Part print with two shaded views. Sizes in mm from the minimum x, y, z corner. A direction names the side the tool comes from. Round coordinates to 2 decimals unless told otherwise and drop trailing zeros. Write each loop counter-clockwise with the first axis right and the second up, starting at its lowest first coordinate (ties: lowest second). Pieces come first, ordered by that corner, then holes. Notation, with made-up numbers: (-31.75, 66) -> (-25.75, 66) arc R22 cw to (-25.75, 88) -> close; hole circle Ø2 at (86, -1.75). An arc over 180 degrees is marked (long way). Return JSON: item names as keys, results as strings. Group by question number.
(1) Saw through at A-A (z = 17.5). List the corners of the cut face in (x, y).
(2) Tool access for the marked faces 1 and 2: list every direction of +Z, -Z, +X, -X, +Y, -Y with a clear straight run to the whole face (end or side of a thin tool).
(3) Drop a flat-ended pin along its axis: pin 1 Ø5 at (x, y) = (178.5, 13) entering from -Z. Give the stop position or say it passes through.
(4) Saw through at C-C (y = 6.5). List the corners of the cut face in (x, z).
(5) Mould opens along Y. For the marked faces 3, 4 and 5 say: +Y half, -Y half, draft (parallel to the pull), parting line (faces both ways), or undercut.
(6) Drill centre lines: L1, parallel to Y at x = 182, z = 36; L2, parallel to X at y = 6, z = 43; L3, parallel to X at y = 35.5, z = 45. Where is each one in solid material? Low to high. Write a range as from..to.
(7) Saw through at B-B (x = 87). List the corners of the cut face in (y, z), plus the area to 3 significant figures.
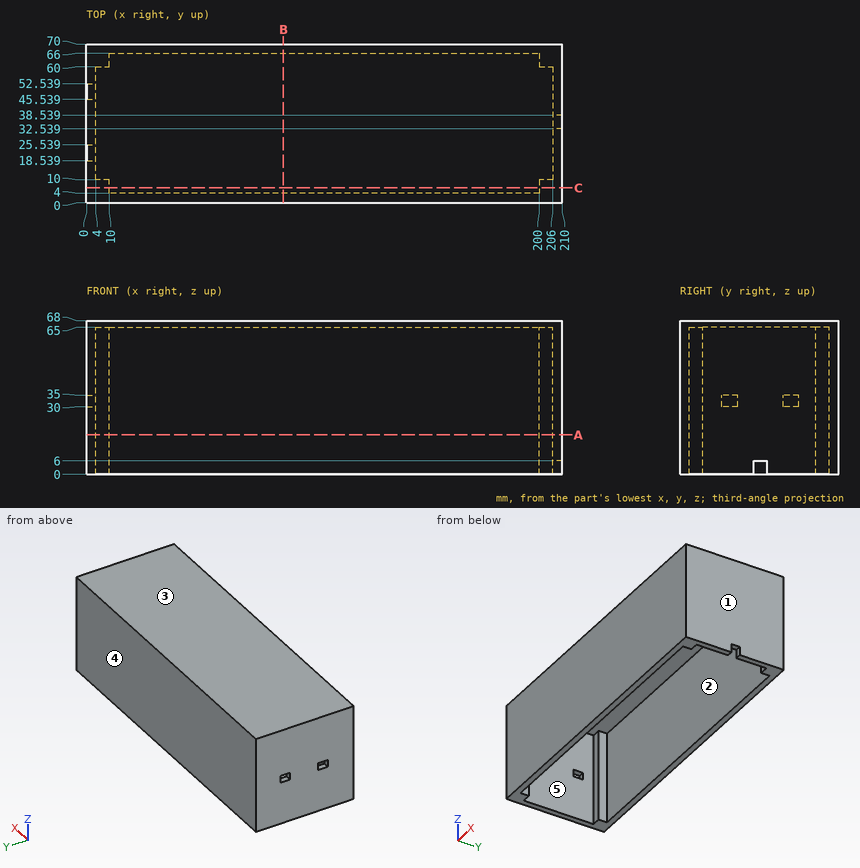
Computed values:
{
 "1": {"outline": "(0, 0) -> (210, 0) -> (210, 70) -> (0, 70) -> close; hole (4, 10) -> (10, 10) -> (10, 4) -> (200, 4) -> (200, 10) -> (206, 10) -> (206, 60) -> (200, 60) -> (200, 66) -> (10, 66) -> (10, 60) -> (4, 60) -> close"},
 "2": {"face 1": "+Z, -Z, +X, +Y, -Y", "face 2": "-Z"},
 "3": {"pin 1": "z = 65"},
 "4": {"outline": "(0, 0) -> (10, 0) -> (10, 65) -> (200, 65) -> (200, 0) -> (210, 0) -> (210, 68) -> (0, 68) -> close"},
 "5": {"face 3": "draft", "face 4": "+Y half", "face 5": "undercut"},
 "6": {"L1": "0..4, 66..70", "L2": "0..10, 200..210", "L3": "0..4, 206..210"},
 "7": {"outline": "(0, 0) -> (4, 0) -> (4, 65) -> (66, 65) -> (66, 0) -> (70, 0) -> (70, 68) -> (0, 68) -> close", "area": "730 mm2"}
}
